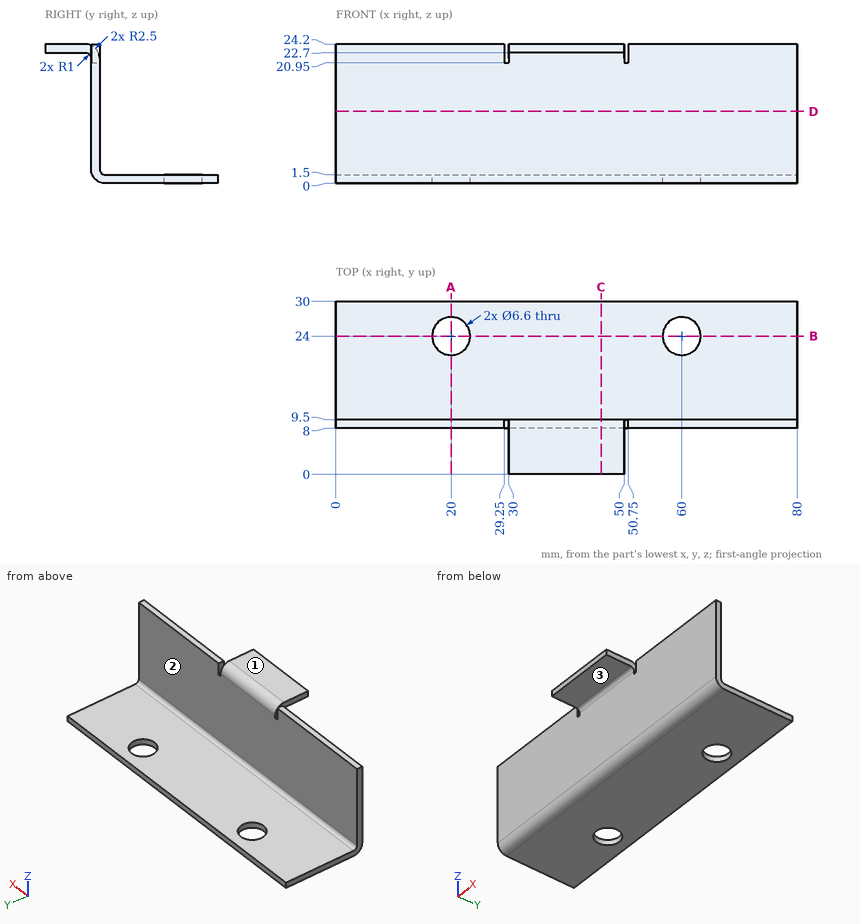
Study the drawing (mm; zero at the part's minimum x, y, z) and answer. A direction names the side the tool comes from. Give positions to 0.01 mm unless a question says otherwise; leave off trailing zeros. Order: outer loops, then holes, each group sorted by start corner. A loop starts at its lowest first (then second) coordinate and runs counter-clockwise, first axis right, second up. Notation, with made-up numbers: (11, 12) - (51, 12) arc R30 cw to (51, 42) - close; hole circle Ø7 at (-34.75, 83.5). An arc over 180 degrees is marked (long way). Answer in a Markdown table with one row per item. Add a question column.
Q1. Given P1, Ø10, axis at x = 27.5, z = 9.5, coming from the -Y side; P2, Ø3.5, axis at y = 3, z = 22, coming from the -X side; P3, Ø8.5, axis at x = 60, y = 24, coming from the +Z side; P4, Ø6, axis at x = 11.5, y = 11.5, coming from the +Z side, each flat-ended and moving along its own axis, determine where each tip first touches the part or whether it passes through.
Q2. Which of the six approach directions +Z, -Z, +X, -X, +Y, -Y give full straight-line access (tool end or side, diameter ignored) to the marked faces 1, 2 and 3?
Q3. Find the intervals of material crossed by line 1 along Z through (x, y) = (4, 15); line 2 along Y through (x, z) = (60, 0.5); line 3 along Y through (x, z) = (49.5, 14.5), in increasing order. Write a range as [from, to].
Q4. The part is cut by section B-B (y = 24). Determine the outline of the cut face in (x, z).
Q5. The part is cut by section C-C (x = 46). Determine the outline of the cut face in (y, z).
Q6. The part is cut by section A-A (x = 20). Determine the outline of the cut face in (y, z).
Q7. The part is cut by section D-D (z = 12.5). Determine the outline of the cut face in (x, y).
Determined:
| question | item | result |
|---|---|---|
| 1 | P1 | stops at y = 8 |
| 1 | P2 | stops at x = 30 |
| 1 | P3 | stops at z = 1.5 |
| 1 | P4 | stops at z = 24.2 |
| 2 | face 1 | +Z, +X, -X, +Y, -Y |
| 2 | face 2 | +Z, +X, -X, +Y |
| 2 | face 3 | -Z, +X, -X, -Y |
| 3 | line 1 | z = [0, 1.5] |
| 3 | line 2 | y = [9, 20.7], [27.3, 30] |
| 3 | line 3 | y = [8, 9.5] |
| 4 | outline | (0, 0) - (16.7, 0) - (16.7, 1.5) - (0, 1.5) - close; (23.3, 0) - (56.7, 0) - (56.7, 1.5) - (23.3, 1.5) - close; (63.3, 0) - (80, 0) - (80, 1.5) - (63.3, 1.5) - close |
| 5 | outline | (0, 22.7) - (7, 22.7) arc R1 cw to (8, 21.7) - (8, 2.5) arc R2.5 ccw to (10.5, 0) - (30, 0) - (30, 1.5) - (10.5, 1.5) arc R1 cw to (9.5, 2.5) - (9.5, 21.7) arc R2.5 ccw to (7, 24.2) - (0, 24.2) - close |
| 6 | outline | (8, 2.5) arc R2.5 ccw to (10.5, 0) - (20.7, 0) - (20.7, 1.5) - (10.5, 1.5) arc R1 cw to (9.5, 2.5) - (9.5, 24.2) - (8, 24.2) - close; (27.3, 0) - (30, 0) - (30, 1.5) - (27.3, 1.5) - close |
| 7 | outline | (0, 8) - (80, 8) - (80, 9.5) - (0, 9.5) - close |
